Here's how the part is built. I have some questions about the finished solid (model axes, mm). Coordinates: 2 decimals unless noted, no trailing zeros. Order: outer loops, then holes, each group sorted by start corner. A loop starts at its lowest first (then second) coordinate and runs counter-clockwise, first axis right, second up. Notation, with made-up numbers: (14.25, -26.5) - (22.25, -26.5) arc R23 ccw to (22.25, -4.5) - close; hole circle Ø5 at (11.25, 32.25). An arc over 180 degrees is marked (long way). Answer in a Markdown table with one row per item. Add a question column.
Item 1: If I drill on line 1 along Z through (x, y) = (-0.5, 6.75); line 2 along X through (y, z) = (0, 205.25); line 3 along Y through (x, z) = (0, 199.75), over which ranges is the centre line in solid material (lowest first)? Write a range as from..to.
Item 2: I want a section at A-A (z = -67). Please give me the cut outline in (x, y).
Item 3: Will these pins go through, and if not, where does the flat tip stop? pin 1 Ø3.5 at (x, y) = (0, 0) entering from +Z; pin 2 Ø1.5 at (y, z) = (4.5, 31) entering from -X; pin 3 Ø4 at (x, z) = (4.5, -111.5) entering from -Y.
```python
from build123d import *

# Parameters (mm, degrees)
BOSS_EXTRUDE1_DEPTH                  = 203.2
SKETCH6_R                            = 6.35
BOSS_EXTRUDE2_DEPTH                  = 7.9375
F_10_32_TAPPED_HOLE1_D               = 4.0386
F_10_32_TAPPED_HOLE1_DEPTH           = 16.34744
F_10_32_TAPPED_HOLE1_TIP             = 1.213317848
F_10_32_TAPPED_HOLE1_ON_FACE_2_D     = 4.0386
F_10_32_TAPPED_HOLE1_ON_FACE_2_DEPTH = 16.34744
F_10_32_TAPPED_HOLE1_ON_FACE_2_TIP   = 1.213317848
SKETCH5_W                            = 0.889
SKETCH5_H                            = 1.0033


with BuildPart() as part:
    # Sketch1 → Boss-Extrude1 (new, symmetric)
    with BuildSketch(Plane.XY):
        with BuildLine():
            ThreePointArc((0.93173274, 6.79441227), (0, 6.858), (-0.93173274, 6.79441227))
            Line((-0.93173274, 6.79441227), (-5.41826726, 4.204110358))
            ThreePointArc((-5.41826726, 4.204110358), (-5.939202219, 3.429), (-6.35, 2.590301913))
            Line((-6.35, 2.590301913), (-6.35, -2.590301913))
            ThreePointArc((-6.35, -2.590301913), (-5.939202219, -3.429), (-5.41826726, -4.204110358))
            Line((-5.41826726, -4.204110358), (-0.93173274, -6.79441227))
            ThreePointArc((-0.93173274, -6.79441227), (0, -6.858), (0.93173274, -6.79441227))
            Line((0.93173274, -6.79441227), (5.41826726, -4.204110358))
            ThreePointArc((5.41826726, -4.204110358), (5.939202219, -3.429), (6.35, -2.590301913))
            Line((6.35, -2.590301913), (6.35, 2.590301913))
            ThreePointArc((6.35, 2.590301913), (5.939202219, 3.429), (5.41826726, 4.204110358))
            Line((5.41826726, 4.204110358), (0.93173274, 6.79441227))
        make_face()
    extrude(amount=BOSS_EXTRUDE1_DEPTH, both=True)

    # Sketch6 → Boss-Extrude2 (add)
    with BuildSketch(Plane.XY.offset(203.2)):
        Circle(SKETCH6_R)
    boss_extrude2 = extrude(amount=BOSS_EXTRUDE2_DEPTH)

    # Mirror2: Boss-Extrude2 across plane
    add(boss_extrude2.mirror(Plane.XY))

    # #10-32 Tapped Hole1
    with Locations(Plane.XY.offset(211.1375)):
        with Locations((0, 0)):
            Hole(F_10_32_TAPPED_HOLE1_D / 2, depth=F_10_32_TAPPED_HOLE1_DEPTH)
            with Locations((0, 0, -(F_10_32_TAPPED_HOLE1_DEPTH + F_10_32_TAPPED_HOLE1_TIP / 2))):  # 118° drill point
                Cone(0, F_10_32_TAPPED_HOLE1_D / 2, F_10_32_TAPPED_HOLE1_TIP, mode=Mode.SUBTRACT)

    # #10-32 Tapped Hole1 on face 2
    with Locations(Plane(origin=(0, 0, -211.1375), x_dir=(-1, 0, 0), z_dir=(0, 0, -1))):
        with Locations((0, 0)):
            Hole(F_10_32_TAPPED_HOLE1_ON_FACE_2_D / 2, depth=F_10_32_TAPPED_HOLE1_ON_FACE_2_DEPTH)
            with Locations((0, 0, -(F_10_32_TAPPED_HOLE1_ON_FACE_2_DEPTH + F_10_32_TAPPED_HOLE1_ON_FACE_2_TIP / 2))):  # 118° drill point
                Cone(0, F_10_32_TAPPED_HOLE1_ON_FACE_2_D / 2, F_10_32_TAPPED_HOLE1_ON_FACE_2_TIP, mode=Mode.SUBTRACT)

    # Sketch5 → Cut-Revolve1 (revolve, cut)
    with BuildSketch(Plane(origin=(0, 0, 0), x_dir=(0, 0, -1), z_dir=(1, 0, 0)), mode=Mode.PRIVATE) as cut_revolve1_sk:
        with Locations((-159.26308, 6.35635)):
            Rectangle(SKETCH5_W, SKETCH5_H)
        with Locations((-145.73758, 6.35635)):
            Rectangle(SKETCH5_W, SKETCH5_H)
    cut_revolve1 = revolve(cut_revolve1_sk.sketch.rotate(Axis((0, 0, 165.047176272), (0, 0, -1)), 90), axis=Axis((0, 0, 165.047176272), (0, 0, -1)), mode=Mode.SUBTRACT)

    # Mirror1: Cut-Revolve1 across plane
    add(cut_revolve1.mirror(Plane.XY), mode=Mode.SUBTRACT)


solid = part.part
```
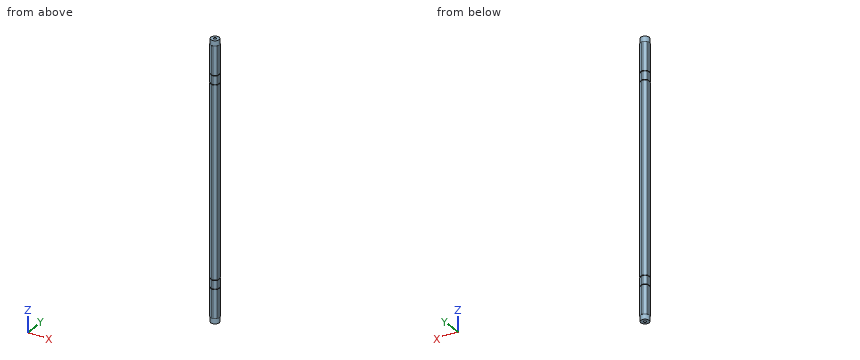
Values follow:
| question | item | result |
|---|---|---|
| 1 | line 1 | z = -203.2..-159.71, -158.82..-146.18, -145.29..145.29, 146.18..158.82, 159.71..203.2 |
| 1 | line 2 | x = -6.35..-2.02, 2.02..6.35 |
| 1 | line 3 | y = -6.86..-2.02, 2.02..6.86 |
| 2 | outline | (-6.35, -2.59) arc R6.86 ccw to (-5.42, -4.2) - (-0.93, -6.79) arc R6.86 ccw to (0.93, -6.79) - (5.42, -4.2) arc R6.86 ccw to (6.35, -2.59) - (6.35, 2.59) arc R6.86 ccw to (5.42, 4.2) - (0.93, 6.79) arc R6.86 ccw to (-0.93, 6.79) - (-5.42, 4.2) arc R6.86 ccw to (-6.35, 2.59) - close |
| 3 | pin 1 | stops at z = 194.63 |
| 3 | pin 2 | stops at x = -5.74 |
| 3 | pin 3 | stops at y = -5.89 |
